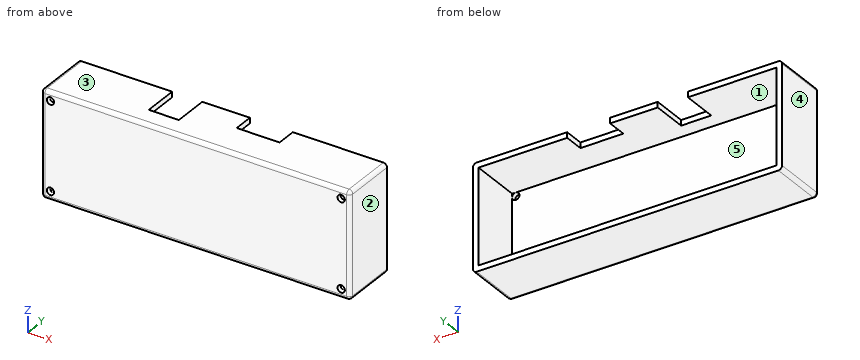
Autodesk Inventor part; units mm, degrees
ref_plane "YZ Plane" through (0, 0, 0) normal (1, 0, 0) x (0, 1, 0)
ref_plane "XZ Plane" through (0, 0, 0) normal (0, 1, 0) x (-1, 0, 0)
ref_plane "XY Plane" through (0, 0, 0) normal (0, 0, 1) x (1, 0, 0)
sketch "Sketch1" plane through (0, 0, 0) normal (0, 1, 0) x (-1, 0, 0)
  line L0 (0, 0) -> (163, 0)
  line L1 (163, 0) -> (163, -52)
  line L2 (163, -52) -> (0, -52)
  line L3 (0, -52) -> (0, 0)
  line L4 (0, 0) -> (-3, 0)
  line L5 (-3, 0) -> (-3, 3)
  line L6 (-3, 3) -> (166, 3)
  line L7 (166, 3) -> (166, -55)
  line L8 (166, -55) -> (-3, -55)
  line L9 (-3, 0) -> (-3, -55)
  dimension "d0" = 163
  dimension "d1" = 52
  dimension "d2" = 3
  dimension "d3" = 3
  dimension "d4" = 169
  dimension "d5" = 58
  dimension "d6" = 169
extrude "Extrusion1" add sketch "Sketch1" along normal blind 28
sketch "Sketch2" plane through (-166, 0, 3) normal (0, 0, 1) x (1, 0, 0)
  line L0 (169, 0) -> (0, 0)
  line L1 (0, 0) -> (169, 0)
  line L2 (169, 0) -> (169, -2.5)
  line L3 (169, -2.5) -> (0, -2.5)
  line L4 (0, -2.5) -> (0, 0)
  point P0 (166, 0)
  dimension "d9" = 2.5
extrude "Extrusion2" add sketch "Sketch2" against normal blind 58
sketch "Sketch3" plane through (-166, 28, 3) normal (0, 0, 1) x (1, 0, 0)
  line L0 (94, 0) -> (117.5, 0)
  line L1 (117.5, 0) -> (117.5, -11)
  line L2 (117.5, -11) -> (94, -11)
  line L3 (94, -11) -> (94, 0)
  line L4 (169, -30.5) -> (169, 0)
  line L5 (0, -30.5) -> (0, 0)
  line L6 (166, -28) -> (3, -28)
  line L7 (0, 0) -> (169, 0)
  line L8 (51.5, -11) -> (68, -11)
  line L9 (68, -11) -> (68, -19.5)
  line L10 (68, -19.5) -> (51.5, -19.5)
  line L11 (51.5, -19.5) -> (51.5, -11)
  line L12 (51.5, -11) -> (68, -19.5) construction
  line L13 (68, -11) -> (51.5, -19.5) construction
  line L14 (0, -30.5) -> (169, -30.5)
  line L15 (51.5, -11) -> (51.5, 0)
  line L16 (68, -11) -> (68, 0)
  line L17 (51.5, 0) -> (68, 0)
  point P0 (59.75, -15.25)
  dimension "d12" = 75
  dimension "d13" = 117.5
  dimension "d14" = 17
  dimension "d15" = 0
  dimension "d16" = 23.5
  dimension "d17" = 16.5
  dimension "d18" = 8.5
  dimension "d19" = 30.5
  dimension "d20" = 15.25
  dimension "d21" = 51.5
  dimension "d22" = 51.5
extrude "Extrusion3" cut sketch "Sketch3" against normal blind 10 contours L0 L1 L2 L3 | L16 L8 L15 L7 | L9 L10 L11 L8
sketch "Sketch4" plane through (-166, -2.5, 3) normal (0, 0, 1) x (1, 0, 0)
  point P0 (166, 2.5)
sketch "Sketch5" plane through (-163, 0, -52) normal (0, 1, 0) x (1, 0, 0)
  circle A0 centre (161, -50) radius 2
  circle A1 centre (161, -2) radius 2
  circle A2 centre (2, -2) radius 2
  circle A3 centre (2, -50) radius 2
  point P0 (163, -52)
  dimension "d25" = 4
  dimension "d26" = 4
  dimension "d27" = 4
  dimension "d28" = 4
  dimension "d29" = 48
  dimension "d30" = 159
extrude "Extrusion4" cut sketch "Sketch5" against normal blind 10
fillet "Fillet1" radius 2 8 edges at (3, 12.75, 3) (3, 12.75, -55) (-166, 12.75, -55) (-166, 12.75, 3) (-81.5, -2.5, -55) (-166, -2.5, -26) (-81.5, -2.5, 3) (3, -2.5, -26)
sketch "Sketch6" plane through (-161, 0, -52) normal (0, 1, 0) x (1, 0, 0)
  line L0 (164, -53) -> (164, 1)
  line L1 (-5, 1) -> (-5, -53)
  line L2 (162, 3) -> (-3, 3)
  line L3 (112.5, -55) -> (162, -55)
  point P0 (161, -52)
  dimension "d34" = 169
  dimension "d35" = 58
sketch "Sketch7" plane through (-98, 28, 3) normal (0, 0, 1) x (1, 0, 0)
  line L0 (49.5, 0) -> (49.5, -11)
  line L1 (101, -28.5) -> (101, 0)
  line L2 (26, -11) -> (49.5, -11)
  line L3 (99, 0) -> (-66, 0)
  line L4 (-68, 0) -> (-68, -28.5)
  line L5 (-16.5, -19.5) -> (-16.5, 0)
  line L6 (0, -19.5) -> (-16.5, -19.5)
  line L7 (26, -11) -> (26, 0)
  point P0 (98, -28)
  dimension "d36" = 51.5
  dimension "d37" = 11
  dimension "d38" = 51.5
  dimension "d39" = 19.5
  dimension "d40" = 23.5
Could you check a few things on this model? Use its own coordinates, in mm. Face numbers are marked on the shaded views. A direction names the side the tool comes from. Round coordinates to 2 decimals unless told otherwise and drop trailing zeros. Order: outer loops, then holes, each group sorted by start corner. A loop starts at its lowest first (then second) coordinate and runs counter-clockwise, first axis right, second up.
(1) Imagine slicing it at A-A (y = 21). Write out the boundary of the cut face in (x, z).
Response values:
outline: (-166, -53) arc R2 ccw to (-164, -55) - (1, -55) arc R2 ccw to (3, -53) - (3, 1) arc R2 ccw to (1, 3) - (-48.5, 3) - (-48.5, 0) - (0, 0) - (0, -52) - (-163, -52) - (-163, 0) - (-114.5, 0) - (-114.5, 3) - (-164, 3) arc R2 ccw to (-166, 1) - close; (-98, 0) - (-72, 0) - (-72, 3) - (-98, 3) - close
(2) Imagine slicing it at B-B (z = -19). Write out the boundary of the cut face in (x, y), plus the area to 3 significant figures.
Response values:
outline: (-166, -0.5) arc R2 ccw to (-164, -2.5) - (1, -2.5) arc R2 ccw to (3, -0.5) - (3, 28) - (0, 28) - (0, 0) - (-163, 0) - (-163, 28) - (-166, 28) - close
area: 589 mm2
(3) Imagine slicing it at C-C (x = -52.5). Write out the boundary of the cut face in (y, z), plus the area to 3 significant figures.
Response values:
outline: (-2.5, -53) arc R2 ccw to (-0.5, -55) - (28, -55) - (28, -52) - (0, -52) - (0, 0) - (17, 0) - (17, 3) - (-0.5, 3) arc R2 ccw to (-2.5, 1) - close
area: 278 mm2
(4) I'm going to push flat-ended pins straight in: pin 1 (0.9 mm diameter, centred on x = -54.5, z = 2, fed in from +Y); pin 2 (1.5 mm diameter, centred on x = -102.5, z = 1.5, fed in from +Y). Where does each tip first touch, or does it pass through?
Response values:
pin 1: stops at y = 17
pin 2: stops at y = 8.5
(5) If we mould it in two halves opening along X, with no side actions, what happens to the marked faces 3, 4 and 5? For each: released by +X, released by -X, zero draft, split by the parting line, or undercut.
Response values:
face 3: zero draft
face 4: released by -X
face 5: undercut
(6) Please list where these lines run through material, in increasing order: line 1 along X through (y, z) = (-0.7, -50); line 2 along X through (y, z) = (22, -50); line 3 along Z through (x, y) = (-161, -0.7).
Response values:
line 1: x = -165.99 to -163, -159 to -4, 0 to 2.99
line 2: x = -166 to -163, 0 to 3
line 3: z = -54.99 to -52, -48 to -4, 0 to 2.99
(7) Which directions (+Z, -Z, +X, -X, +Y, -Y) give clear straight access to the entire face, cutting with the end or side of a thin tool? Please do the marked faces 1 and 2.
Response values:
face 1: +Y
face 2: +Z, -Z, +X, +Y, -Y
(8) Imagine slicing it at D-D (y = 2). Write out the boundary of the cut face in (x, z).
Response values:
outline: (-166, -53) arc R2 ccw to (-164, -55) - (1, -55) arc R2 ccw to (3, -53) - (3, 1) arc R2 ccw to (1, 3) - (-164, 3) arc R2 ccw to (-166, 1) - close; hole (-163, -52) - (0, -52) - (0, 0) - (-163, 0) - close
